Can you work these out from the model? Positions are in its coordinate system, mm. A direction names the side the tool comes from. Round coordinates to 2 decimals unless told otherwise and drop trailing zeros. Write each loop counter-clockwise with the first axis right and the second up, starting at its lowest first coordinate (ties: lowest second). Pieces come first, ordered by that corner, then holes. Notation, with made-up numbers: (37.5, 37) - (47.5, 37) arc R5 cw to (47.5, 45) - close; hole circle Ø2 at (40.5, 22). An arc over 180 degrees is marked (long way). One line per item, written item: value. Start each with the question number.
(1) I want a section at A-A on y = 2.5. List the corners of the cut face in (x, z) for me (3 decimals), plus the area to 3 significant figures.
(2) On a 3-axis mill with a long thin cutter (end or side, diameter ignored), from which of +Z, -Z, +X, -X, +Y, -Y can I reach the whole of each face in a straight line? I mean faces 4 (the face through (-6, -0.5, 4)), 5 (the face through (-6.694, 2.718, 0.295)), 6 (the face through (-7.75, 2.47, -2.44)). Say none if no direction works.
(3) I'm going to push flat-ended pins straight in: pin 1 Ø4 at (x, z) = (-5.5, 0.5) entering from -Y; pin 2 Ø4 at (x, y) = (-6, 2) entering from +Z; pin 3 Ø4 at (y, z) = (1, 6) entering from +X. Where does each tip first touch, or does it pass through?
(4) Thinking about a two-plate mould opening in X: for faces 1 (the face through (9, -5, -1)), 2 (the face through (7.638, -4.683, -5.857)), 3 (the face through (3, 0.5, -7)), which applies, +X half, -X half, draft (parallel to the pull), parting line (faces both ways), or undercut?
(5) I want a section at B-B on y = -2.5. List the corners of the cut face in (x, z) for me (3 decimals).
(6) If I drill on L1, parallel to Z at x = 0, y = 1.55 (3 decimals); L2, parallel to Z at x = 0, y = -0.1; L3, parallel to Z at x = -4.5, y = 3.75, over which ranges is the centre line in solid material (lowest first)? Write a range as from..to.
Autodesk Inventor part; units mm, degrees
ref_plane "YZ Plane" through (0, 0, 0) normal (1, 0, 0) x (0, 1, 0)
ref_plane "XZ Plane" through (0, 0, 0) normal (0, 1, 0) x (-1, 0, 0)
ref_plane "XY Plane" through (0, 0, 0) normal (0, 0, 1) x (1, 0, 0)
sketch "Sketch1" plane through (0, 0, 0) normal (0, 0, 1) x (1, 0, 0)
  line L0 (0, -0.4401) -> (0, 0.4401)
  line L1 (-8.125, -0.5) -> (-6.95, -0.5)
  line L2 (-6.95, -0.5) -> (-6.95, 0.5)
  line L3 (-6.95, 0.5) -> (-8.125, 0.5)
  line L4 (-8.125, 0.5) -> (-8.125, -0.5)
  line L5 (-8.125, -0.5) -> (-6.95, 0.5) construction
  line L6 (-6.95, -0.5) -> (-8.125, 0.5) construction
  line L7 (-9.625, 5) -> (-8.125, 5)
  line L8 (-8.125, 5) -> (-8.125, -5)
  line L9 (-8.125, -5) -> (-9.625, -5)
  line L10 (-9.625, -5) -> (-9.625, 5)
  line L11 (-9.625, 5) -> (-8.125, -5) construction
  line L12 (-8.125, 5) -> (-9.625, -5) construction
  line L13 (-9.625, -4.375) -> (-12, -2)
  line L14 (-12, -2) -> (-12, 2)
  line L15 (-12, 2) -> (-9.625, 4.375)
  line L16 (-8, 0.5) -> (8, 0.5) construction
  line L17 (8, 0.5) -> (8, 5.5) construction
  line L18 (8, 5.5) -> (-8, 5.5) construction
  line L19 (-8, 5.5) -> (-8, 0.5) construction
  line L20 (-8, 0.5) -> (8, 5.5) construction
  line L21 (8, 0.5) -> (-8, 5.5) construction
  line L22 (-17, -3) -> (-11, -3) construction
  line L23 (-11, -3) -> (-11, 3) construction
  line L24 (-11, 3) -> (-17, 3) construction
  line L25 (-17, 3) -> (-17, -3) construction
  line L26 (-17, -3) -> (-11, 3) construction
  line L27 (-11, -3) -> (-17, 3) construction
  point P0 (0, 0)
  point P1 (0, 0)
  point P2 (-7.5375, 0)
  point P3 (-8.875, 0)
  point P4 (-12, 0)
  point P5 (-7.5375, 0)
  point P6 (-8.875, 0)
  point P7 (0, 3)
  point P8 (0, 3)
  point P9 (-14, 0)
  point P10 (-8.125, 0.5)
  point P11 (-8.125, -0.5)
  dimension "d0" = 13.9
  dimension "d1" = 16.25
  dimension "d2" = 10
  dimension "d3" = 16
  dimension "d4" = 5
  dimension "d5" = 5.5
  dimension "d6" = 45
  dimension "d7" = 4
  dimension "d8" = 2.375
  dimension "d9" = 1.5
  dimension "d10" = 6
  dimension "d11" = 6
  dimension "d12" = 22
revolve "Revolution1" add sketch "Sketch1" angle 360 about axis through (0, -0.4401, 0) along (0, 1, 0)
chamfer "Chamfer1" distance 0.5 angle 45 2 edges at (8.125, 5, 0) (8.125, -5, 0)
sketch "Sketch2" plane through (0, 0.5, 0) normal (0, 1, 0) x (1, 0, 0)
  circle A0 centre (0, 0) radius 6.95 construction
  circle A1 centre (0, 0) radius 7.2
  circle A2 centre (0, 0) radius 6.7
  point P0 (0, 0)
  dimension "d17" = 0.25
  dimension "d18" = 0.25
extrude "Extrusion1" add sketch "Sketch2" along normal up to surface (4.5 mm away)
properties part number "Internal_V-groove_Bearing"
Established:
1. outline: circle Ø23 at (0, 0); circle Ø14.4 at (0, 0); hole circle Ø16.25 at (0, 0); hole circle Ø13.4 at (0, 0)
1. area: 230 mm2
2. face 4: -Y
2. face 5: +Y, -Y
2. face 6: +Y
3. pin 1: y = -0.5
3. pin 2: z = 11.31
3. pin 3: x = 11.31
4. face 1: draft
4. face 2: parting line
4. face 3: undercut
5. outline: circle Ø23 at (0, 0); hole circle Ø16.25 at (0, 0)
6. L1: -12..-8.125, -7.2..-6.7, 6.7..7.2, 8.125..12
6. L2: -12..-6.95, 6.95..12
6. L3: -9.21..-6.77, -5.62..-4.96, 4.96..5.62, 6.77..9.21
